```python
from build123d import *

# Parameters (mm, degrees)
SKETCH1_W           = 533.4
SKETCH1_H           = 635
BOSS_EXTRUDE1_DEPTH = 76.2
SKETCH2_W           = 508
SKETCH2_H           = 609.6
CUT_EXTRUDE1_DEPTH  = 422.594093887
FILLET1_R           = 6.35


with BuildPart() as part:
    # Sketch1 → Boss-Extrude1 (new body)
    with BuildSketch(Plane.XY):
        Rectangle(SKETCH1_W, SKETCH1_H)
    extrude(amount=BOSS_EXTRUDE1_DEPTH)

    # Sketch2 → Cut-Extrude1 (cut, through all)
    with BuildSketch(Plane.XY.offset(76.2)):
        Rectangle(SKETCH2_W, SKETCH2_H)
    extrude(amount=-CUT_EXTRUDE1_DEPTH, mode=Mode.SUBTRACT)

    # Fillet1
    fillet1_edges = [part.edges().sort_by_distance(p)[0] for p in [
        (266.7, -317.5, 38.1),
        (-266.7, -317.5, 38.1),
        (-266.7, 317.5, 38.1),
        (266.7, 317.5, 38.1),
    ]]
    fillet(fillet1_edges, radius=FILLET1_R)


solid = part.part
```
Verification items for the finished model (mm, model axes). A direction names the side the tool comes from. Give positions to 0.01 mm unless a question says otherwise; leave off trailing zeros. Write each loop counter-clockwise with the first axis right and the second up, starting at its lowest first coordinate (ties: lowest second). Pieces come first, ordered by that corner, then holes. Notation, with made-up numbers: M 67.25,71 L 76.25,71 A16 ccw 76.25,79 Z; hole C -31.5,-22.75 d3. An arc over 180 degrees is marked long. One line per question, with ' | ' between items.
1) Thickness scan on line 1 along Y through (x, z) = (-111, 36); line 2 along X through (y, z) = (222, 19). Record the ranges inside material, lowest first. Write a range as [from, to].
Result:
line 1: y = [-317.5, -304.8], [304.8, 317.5] | line 2: x = [-266.7, -254], [254, 266.7]
2) Section check A-A on x = 82. Enter the section's corners in (y, z).
Result:
outline: M -317.5,0 L -304.8,0 L -304.8,76.2 L -317.5,76.2 Z; M 304.8,0 L 317.5,0 L 317.5,76.2 L 304.8,76.2 Z
3) Section check B-B on y = 90.5. Enter the section's corners in (x, z).
Result:
outline: M -266.7,0 L -254,0 L -254,76.2 L -266.7,76.2 Z; M 254,0 L 266.7,0 L 266.7,76.2 L 254,76.2 Z
4) Mould release check, pull along Y, two halves, no side actions. Record for faces 1 (the flat face through (-1, 307, 76.2)), 2 (the flat face through (-4, -317.5, 38)), 3 (the flat face through (-4, -304.8, 39)): released by +Y, released by -Y, zero draft, split by the parting line, or undercut.
Result:
face 1: zero draft | face 2: released by -Y | face 3: undercut
5) Set-up check for faces 4 (the flat face through (-266.7, -4, 38)), 5 (the flat face through (-254, -4, 39)): record each of +Z, -Z, +X, -X, +Y, -Y from which the full face is reachable in a straight line by a thin tool's end or side.
Result:
face 4: +Z, -Z, -X, +Y, -Y | face 5: +Z, -Z
6) Section check C-C on z = 34. Enter the section's corners in (x, y).
Result:
outline: M -266.7,-311.15 A6.35 ccw -260.35,-317.5 L 260.35,-317.5 A6.35 ccw 266.7,-311.15 L 266.7,311.15 A6.35 ccw 260.35,317.5 L -260.35,317.5 A6.35 ccw -266.7,311.15 Z; hole M -254,-304.8 L 254,-304.8 L 254,304.8 L -254,304.8 Z
